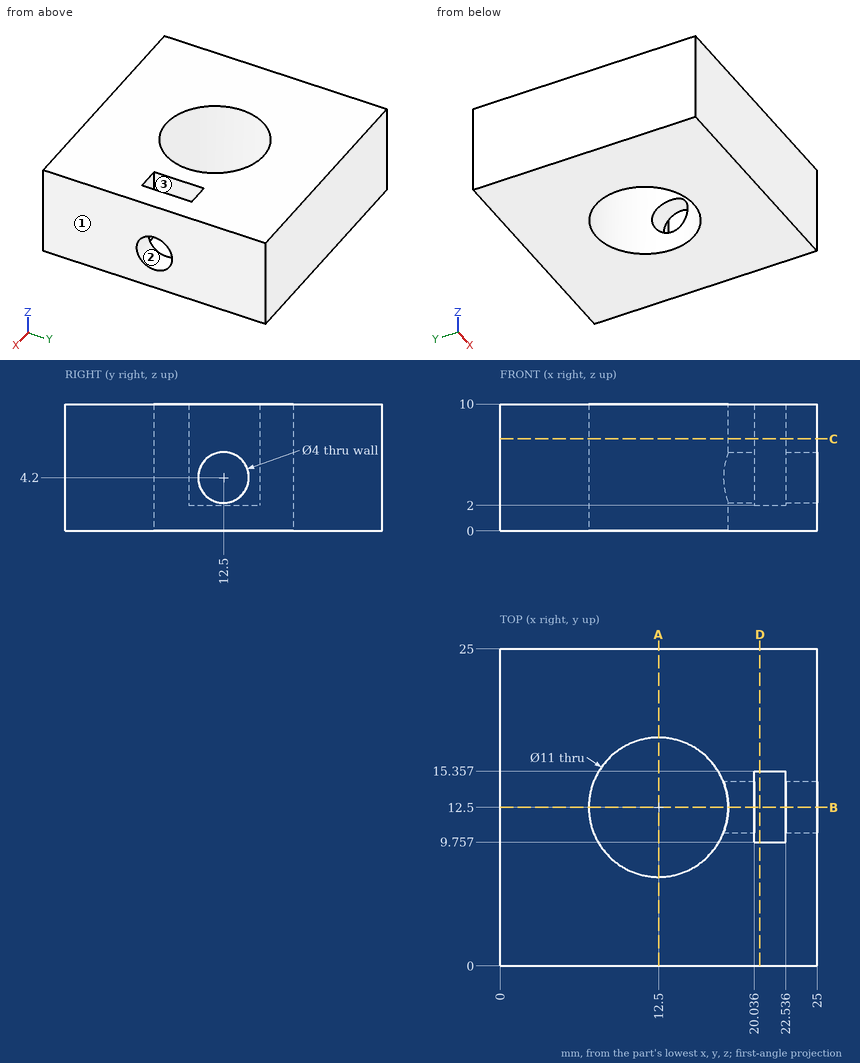
Print and shaded views of the part. All mm, measured from the part's lowest x, y and z. Give positions to 0.01 mm unless a question says otherwise; leave off trailing zeros. Loops run counter-clockwise (first coordinate to the right, second up) from the corner with the lowest first, then second, coordinate; pieces in that order, holes last. Notation, with made-up numbers: (-24.75, 63.5) -> (5.25, 63.5) arc R15 cw to (5.25, 69.5) -> close; hole circle Ø5 at (20, -17.5). An arc over 180 degrees is marked (long way). Answer in a Markdown table with one row per item.
Item 1: Slice it at D-D on x = 20.5. Write the cut outline in (y, z), plus the area to 3 significant figures.
Findings below:
| item | result |
|---|---|
| outline | (0, 0) -> (25, 0) -> (25, 10) -> (15.36, 10) -> (15.36, 2) -> (9.76, 2) -> (9.76, 10) -> (0, 10) -> close |
| area | 205 mm² |
Item 2: Mould opens along X. For the marked faces 1, 2 and 3 say: pulls with the +X half, pulls with the -X half, needs draft (parallel to the pull), parting line crosses it, or undercut.
Findings below:
| item | result |
|---|---|
| face 1 | pulls with the +X half |
| face 2 | needs draft |
| face 3 | undercut |
Item 3: Slice it at A-A on x = 12.5. Write the cut outline in (y, z), plus the area to 3 significant figures.
Findings below:
| item | result |
|---|---|
| outline | (0, 0) -> (7, 0) -> (7, 10) -> (0, 10) -> close; (18, 0) -> (25, 0) -> (25, 10) -> (18, 10) -> close |
| area | 140 mm² |
Item 4: Slice it at C-C on z = 7.25. Write the cut outline in (x, y).
Findings below:
| item | result |
|---|---|
| outline | (0, 0) -> (25, 0) -> (25, 25) -> (0, 25) -> close; hole circle Ø11 at (12.5, 12.5); hole (20.04, 9.76) -> (22.54, 9.76) -> (22.54, 15.36) -> (20.04, 15.36) -> close |
Item 5: Slice it at B-B on y = 12.5. Write the cut outline in (x, z), plus the area to 3 significant figures.
Findings below:
| item | result |
|---|---|
| outline | (0, 0) -> (7, 0) -> (7, 10) -> (0, 10) -> close; (18, 0) -> (25, 0) -> (25, 2.2) -> (22.54, 2.2) -> (22.54, 2) -> (20.04, 2) -> (20.04, 2.2) -> (18, 2.2) -> close; (18, 6.2) -> (20.04, 6.2) -> (20.04, 10) -> (18, 10) -> close; (22.54, 6.2) -> (25, 6.2) -> (25, 10) -> (22.54, 10) -> close |
| area | 102 mm² |
Item 6: Flat gauge pins, fed straight in: P1, Ø9, axis at x = 12.5, y = 12.5, coming from the +Z side; P2, Ø1.2, axis at x = 21.5, y = 13, coming from the +Z side. Where does each tip first touch, or does it go through?
Findings below:
| item | result |
|---|---|
| P1 | passes through |
| P2 | stops at z = 2 |
Item 7: Probe line 1 along Y through (x, z) = (21.25, 5); line 2 along Y through (x, z) = (12.5, 5.5); line 3 along X through (y, z) = (10.25, 7.5). List the from-to ranges inside material, lowest first. Write a range as [from, to].
Findings below:
| item | result |
|---|---|
| line 1 | y = [0, 9.76], [15.36, 25] |
| line 2 | y = [0, 7], [18, 25] |
| line 3 | x = [0, 7.48], [17.52, 20.04], [22.54, 25] |
